The listing builds one solid part. Answer for the finished solid, in the listing's coordinates (mm). Face numbers are marked on the shaded views. A direction names the side the tool comes from. Round coordinates to 2 decimals unless told otherwise and drop trailing zeros. Loops run counter-clockwise (first coordinate to the right, second up) from the corner with the lowest first, then second, coordinate; pieces in that order, holes last. Notation, with made-up numbers: (62.5, 34.5) - (103.5, 34.5) arc R28 ccw to (103.5, 70.5) - close; hole circle Ø2 at (64.25, -4.5). An arc over 180 degrees is marked (long way). Write item = value, one per line. Start each with the question number.
1) Section D-D, the plane y = 5.5 is taken. Determine the outline of the cut face in (x, z).
2) Section B-B, the plane z = 7 is taken. Determine the outline of the cut face in (x, y).
3) Section A-A, the plane x = -0.5 is taken. Determine the outline of the cut face in (y, z), and give its area (3 significant figures).
4) Section C-C, the plane z = 4.5 is taken. Determine the outline of the cut face in (x, y), and give its area (3 significant figures).
5) A tool of negligible diameter and unlimited length cuts with its end or side. For the marked faces 1, 2, 3 and 4, from which of +Z, -Z, +X, -X, +Y, -Y can it reach the whole face along a straight path? Write none if from no direction.
6) Straight lines are drawn through the part: line 1 along Y through (x, z) = (-1.5, 6); line 2 along X through (y, z) = (-6.5, 4.25); line 3 along Z through (x, y) = (-1, 2). For each, find the intervals that lie inside material, in ascending order.
7) Given pin 1 Ø3 at (x, y) = (-2.5, 2) entering from -Z; pin 2 Ø1.5 at (x, z) = (-4.5, 2) entering from -Y; pin 3 Ø1 at (x, z) = (2, 6.5) entering from -Y, each flat-ended and moving along its own axis, determine where each tip first touches the part or whether it passes through.
from build123d import *

# Parameters (mm, degrees)
F0_W          = 5.15
F0_H          = 11
F1_DEPTH      = 14
F3_DEPTH      = 5.151
F3_DEPTH_BACK = 5.151
F5_DEPTH      = 1.75
F6_R          = 6
F7_T4_DEPTH   = 15.5
F7_T9_DEPTH   = 15.5
F8_R          = 0.5


# Not quite as in the source:
# - a fillet or chamfer that OpenCascade refuses, or shapes differently, is made with other operations: its cross-section is extruded or revolved along the edge and cut away or added


with BuildPart() as f1:
    # F0 (on Front) → F1 (new body)
    with BuildSketch(Plane.XZ):
        with Locations((2.575, 0)):
            Rectangle(F0_W, F0_H)
        Polygon((0, 5.5), (5.15, 5.5), (2.5, 10), (0, 10), align=None)
        with Locations((-2.575, 0)):
            Rectangle(F0_W, F0_H)
        Polygon((-5.15, 5.5), (0, 5.5), (0, 10), (-2.5, 10), align=None)
    extrude(amount=-F1_DEPTH)

    # F2 (on Right) → F3 (cut, two sides)
    with BuildSketch(Plane.YZ) as f3_sk:
        with BuildLine():
            Line((4.0006404915, 10), (4.0006404915, 5.5))
            ThreePointArc((4.0006404915, 5.5), (7.2844648336, 2.2498275803), (10.5006404915, 5.5669554351))
            Line((10.5006404915, 5.5669554351), (10.5, 10))
            Line((10.5, 10), (4.0006404915, 10))
        make_face()
    extrude(amount=F3_DEPTH, mode=Mode.SUBTRACT)
    extrude(f3_sk.sketch, amount=-F3_DEPTH_BACK, mode=Mode.SUBTRACT)

    # F4 (on Right) → F5 (join, symmetric)
    with BuildSketch(Plane.YZ):
        Polygon((0, -9.5), (0, 0), (0, 14), (-3.5, 14), (-18.5, 8), (-18.5, -4.5), (-3.5, -9.5), align=None)
    extrude(amount=F5_DEPTH, both=True)

    # F6
    f6_edges = [f1.edges().sort_by_distance(p)[0] for p in [
        (0, 14, -5.5),
    ]]
    fillet(f6_edges, radius=F6_R)

    # F7: fillet of radius 2 on 2 edges, made by hand


with BuildPart() as f7_tool2:
    # F7_s3 → F7_t4 (new body)
    with BuildSketch(Plane.XY.offset(10)):
        with BuildLine():
            ThreePointArc((3.75, 0), (2.3357864376, -0.5857864376), (1.75, -2))
            Line((1.75, -2), (1.75, 0))
            Line((1.75, 0), (3.75, 0))
        make_face()
    extrude(amount=-F7_T4_DEPTH)

    split(bisect_by=Plane(origin=(6.2288019067, 0, 3.6680722339), x_dir=(0, 1, 0), z_dir=(-0.8616879874, 0, -0.5074384814)), keep=Keep.TOP)


with BuildPart() as f1_1:
    add(f1.part)

    # F7_t1: union F7_tool2
    add(f7_tool2.part)


with BuildPart() as f7_tool7:
    # F7_s8 → F7_t9 (new body)
    with BuildSketch(Plane.XY.offset(-5.5)):
        with BuildLine():
            ThreePointArc((-3.75, 0), (-2.3357864376, -0.5857864376), (-1.75, -2))
            Line((-1.75, -2), (-1.75, 0))
            Line((-1.75, 0), (-3.75, 0))
        make_face()
    extrude(amount=F7_T9_DEPTH)

    split(bisect_by=Plane(origin=(-6.2288019067, 0, 3.6680722339), x_dir=(0, 1, 0), z_dir=(0.8616879874, 0, -0.5074384814)), keep=Keep.TOP)


with BuildPart() as f1_2:
    add(f1_1.part)

    # F7_t6: union F7_tool7
    add(f7_tool7.part)

    # F8
    f8_edges = [f1_2.edges().sort_by_distance(p)[0] for p in [
        (1.75, -11, 11),
        (1.75, -1.75, 14),
        (1.75, -18.5, 1.75),
        (1.75, -11, -7),
        (1.75, -1.75, -9.5),
        (-1.75, -11, 11),
        (-1.75, -1.75, 14),
        (-1.75, -11, -7),
    ]]
    fillet(f8_edges, radius=F8_R)


solid = f1_2.part
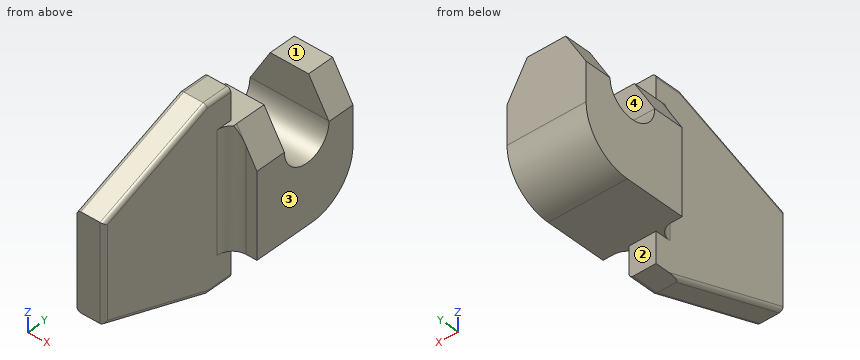
Geometry check:
q1.outline = (-5.15, -5.5) - (5.15, -5.5) - (5.15, 2.76) - (-5.15, 2.76) - close
q2.outline = (-4.27, 0) - (-3.75, 0) arc R2 cw to (-1.75, -2) - (-1.75, -18.5) - (1.25, -18.5) arc R0.5 ccw to (1.75, -18) - (1.75, -2) arc R2 cw to (3.75, 0) - (4.27, 0) - (4.27, 4) - (-4.27, 4) - close; (-4.27, 10.5) - (4.27, 10.5) - (4.27, 14) - (-4.27, 14) - close
q3.outline = (-18.5, -4.5) - (-3.5, -9.5) - (0, -9.5) - (0, -5.5) - (8, -5.5) arc R6 ccw to (14, 0.5) - (14, 10) - (10.5, 10) - (10.5, 5.57) arc R3.25 cw (long way) to (4, 5.5) - (4, 10) - (0, 10) - (0, 14) - (-3.5, 14) - (-18.5, 8) - close
q3.area = 516 mm2
q4.outline = (-5.15, 0) - (-3.75, 0) arc R2 cw to (-1.75, -2) - (-1.75, -18.5) - (1.25, -18.5) arc R0.5 ccw to (1.75, -18) - (1.75, -2) arc R2 cw to (3.75, 0) - (5.15, 0) - (5.15, 4.16) - (-5.15, 4.16) - close; (-5.15, 10.34) - (5.15, 10.34) - (5.15, 14) - (-5.15, 14) - close
q4.area = 147 mm2
q5.face_1 = +Z, +X, -X, +Y
q5.face_2 = -Z, +X, -X, +Y
q5.face_3 = +Z, -Z, +X, +Y, -Y
q5.face_4 = +Z, +X, -X
q6.line_1 = -18.5 to 4, 10.5 to 14
q6.line_2 = -1.75 to 1.75
q6.line_3 = -5.5 to 10
q7.pin_1 = -5.5
q7.pin_2 = 0
q7.pin_3 = -18.43
